Could you check a few things on this drawing? It's one solid part, dimensions in mm from its lowest x, y, z. Round coordinates to 2 decimals unless told otherwise and drop trailing zeros. Write each loop counter-clockwise with the first axis right and the second up, starting at its lowest first coordinate (ties: lowest second). Pieces come first, ordered by that corner, then holes. Notation, with made-up numbers: (11.25, 67.25) -> (20.25, 67.25) arc R16 ccw to (20.25, 83.25) -> close; hole circle Ø10 at (15, -36). An arc over 180 degrees is marked (long way). Answer in a Markdown table with one row per item. Add a question column.
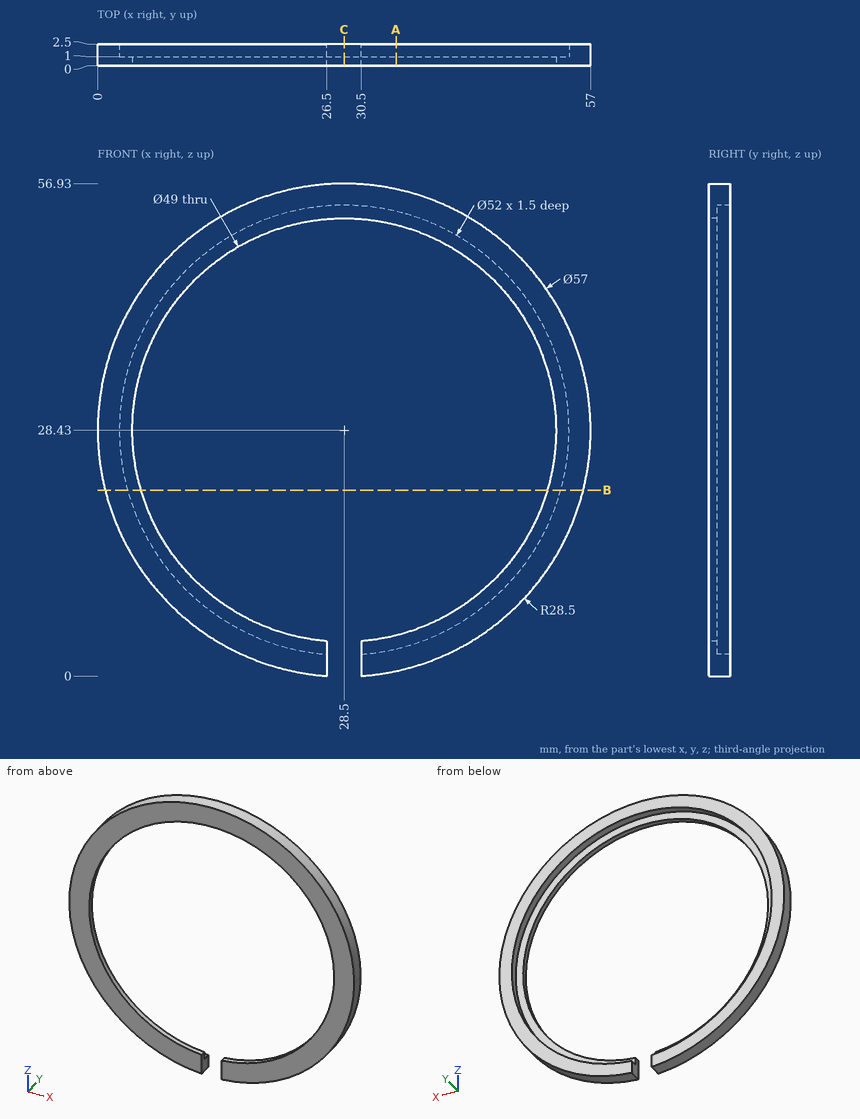
Item 1: If we section it at C-C on x = 28.5: Please give me the cut outline in (y, z).
Item 2: If we section it at B-B on z = 21.5: Please give me the cut outline in (x, y) (1 decimal).
Item 3: I need wall thicknesses on line 1 along Z through (x, y) = (28.5, 0.4); line 2 along X through (y, z) = (0.45, 10.5) (1 decimal); line 3 along Z through (x, y) = (25, 2.35) (1 decimal). Which ranges of each line are inside material? Lowest first, please. Write a range as from..to.
Item 4: For P1, Ø3, axis at x = 15.5, z = 9.5, coming from the -Y side; P2, Ø1.5, axis at y = 2, z = 22, coming from the +X side, each with a flat end and sliding along its axis, tell me the tip position at first contact or that it passes through.
Item 5: If we section it at A-A on x = 34.5: Please give me the cut outline in (y, z).
Results list:
| question | item | result |
|---|---|---|
| 1 | outline | (0, 52.93) -> (1, 52.93) -> (1, 54.43) -> (2.5, 54.43) -> (2.5, 56.93) -> (0, 56.93) -> close |
| 2 | outline | (0.9, 0) -> (5, 0) -> (5, 1) -> (3.4, 1) -> (3.4, 2.5) -> (0.9, 2.5) -> close; (52, 0) -> (56.1, 0) -> (56.1, 2.5) -> (53.6, 2.5) -> (53.6, 1) -> (52, 1) -> close |
| 3 | line 1 | 52.93..56.93 |
| 3 | line 2 | 6.3..11.8, 45.2..50.7 |
| 3 | line 3 | 0.1..2.7, 54.2..56.7 |
| 4 | P1 | through |
| 4 | P2 | x = 56.43 |
| 5 | outline | (0, 0.57) -> (2.5, 0.57) -> (2.5, 3.13) -> (1, 3.13) -> (1, 4.68) -> (0, 4.68) -> close; (0, 52.18) -> (1, 52.18) -> (1, 53.73) -> (2.5, 53.73) -> (2.5, 56.29) -> (0, 56.29) -> close |
